Here's the drawing with two shaded views (mm, measured from the low corner). I have some questions. A direction names the side the tool comes from. Round coordinates to 2 decimals unless told otherwise and drop trailing zeros. Order: outer loops, then holes, each group sorted by start corner. A loop starts at its lowest first (then second) coordinate and runs counter-clockwise, first axis right, second up. Notation, with made-up numbers: (-14, -6) -> (-5, -6) arc R21 cw to (-5, 23) -> close; hole circle Ø4 at (34, -36.5). An arc over 180 degrees is marked (long way). Answer in a Markdown table with one row per item.
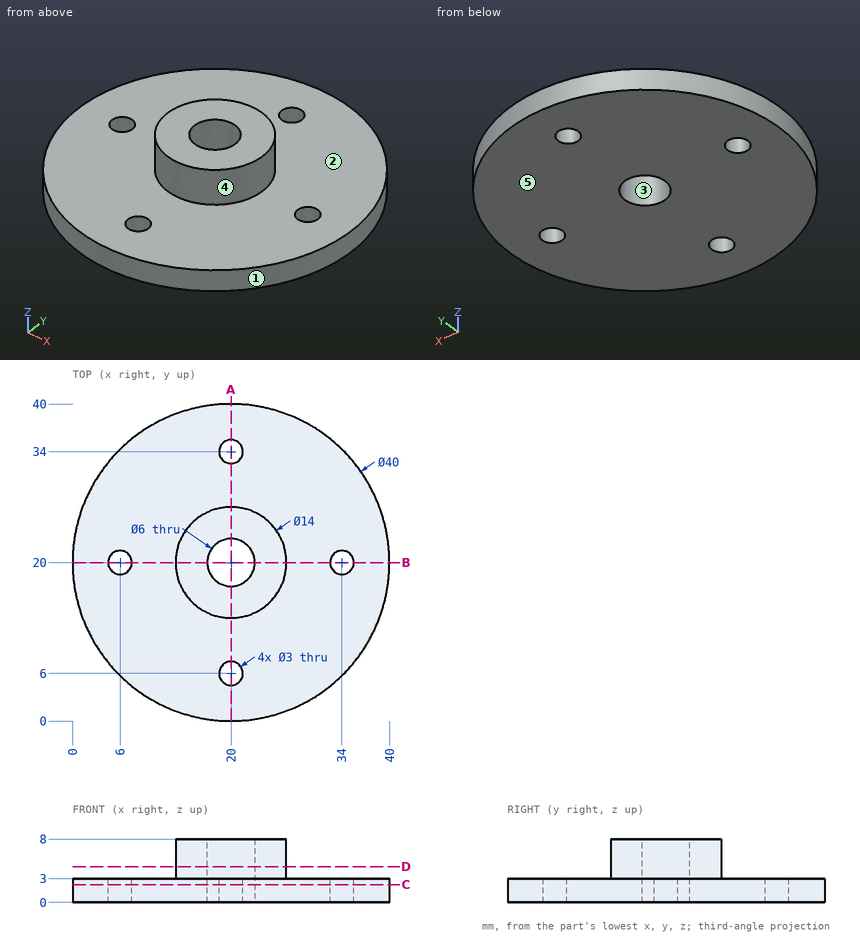
1. For pin 1 Ø3.5 at (x, y) = (6, 20) entering from +Z; pin 2 Ø3 at (y, z) = (29, 4) entering from +X; pin 3 Ø4 at (y, z) = (6.5, 2.5) entering from +X, each with a flat end and sliding along its axis, tell me the tip position at first contact or that it passes through.
Numbers:
| item | result |
|---|---|
| pin 1 | stops at z = 3 |
| pin 2 | stops at x = 38.38 |
| pin 3 | stops at x = 36.36 |
2. Please list where these lines run through material, in increasing order: line 1 along Y through (x, z) = (20, 2); line 2 along Z through (x, y) = (19.5, 38); line 3 along X through (y, z) = (34, 2.05).
Numbers:
| item | result |
|---|---|
| line 1 | y = 0 to 4.5, 7.5 to 17, 23 to 32.5, 35.5 to 40 |
| line 2 | z = 0 to 3 |
| line 3 | x = 5.72 to 18.5, 21.5 to 34.28 |
3. Suppose I cut it at D-D on z = 4.5. Write out the boundary of the cut face in (x, y), then the cut area to 3 significant figures.
Numbers:
| item | result |
|---|---|
| outline | circle Ø14 at (20, 20); hole circle Ø6 at (20, 20) |
| area | 126 mm2 |
4. Suppose I cut it at A-A on x = 20. Write out the boundary of the cut face in (y, z).
Numbers:
| item | result |
|---|---|
| outline | (0, 0) -> (4.5, 0) -> (4.5, 3) -> (0, 3) -> close; (7.5, 0) -> (17, 0) -> (17, 8) -> (13, 8) -> (13, 3) -> (7.5, 3) -> close; (23, 0) -> (32.5, 0) -> (32.5, 3) -> (27, 3) -> (27, 8) -> (23, 8) -> close; (35.5, 0) -> (40, 0) -> (40, 3) -> (35.5, 3) -> close |
5. We'd pull the mould along Y, two halves only. Please class the marked faces 1, 2 and 3: released by +Y, released by -Y, zero draft, split by the parting line, or undercut.
Numbers:
| item | result |
|---|---|
| face 1 | split by the parting line |
| face 2 | zero draft |
| face 3 | undercut |
6. Suppose I cut it at C-C on z = 2.25. Write out the boundary of the cut face in (x, y), then the cut area to 3 significant figures.
Numbers:
| item | result |
|---|---|
| outline | circle Ø40 at (20, 20); hole circle Ø3 at (6, 20); hole circle Ø6 at (20, 20); hole circle Ø3 at (20, 6); hole circle Ø3 at (20, 34); hole circle Ø3 at (34, 20) |
| area | 1,200 mm2 |
7. For the marked faces 4 and 5, which set-ups out of +Z, -Z, +X, -X, +Y, -Y let a thin tool reach every point of the face, with its end or its side?
Numbers:
| item | result |
|---|---|
| face 4 | +Z |
| face 5 | -Z, +X, -X, +Y, -Y |
